Here's how the part is built. I have some questions about the finished solid (model axes, mm). A direction names the side the tool comes from. Round coordinates to 2 decimals unless told otherwise and drop trailing zeros. Write each loop counter-clockwise with the first axis right and the second up, starting at its lowest first coordinate (ties: lowest second). Pieces come first, ordered by that corner, then holes. Notation, with made-up numbers: (-12, -3.5) -> (41, -3.5) arc R22 ccw to (41, 6.5) -> close; hole circle Ø1 at (12.5, 73). An arc over 180 degrees is marked (long way). Put each result on its own line as item: value. Start each with the question number.
1) I want a section at B-B, the plane z = 25. List the corners of the cut face in (x, y) for me.
2) Which directions (+Z, -Z, +X, -X, +Y, -Y) give clear straight access to the entire face, cutting with the end or side of a thin tool? Please do faces 4 (the cylindrical face through (-0.03, 0.24, 35.64)), 5 (the conical face through (0.047, 2.147, 33.856)), 6 (the flat face through (1.9, 0, 33.9)), 7 (the cylindrical face through (-2.539, -1.947, 0.74)), 8 (the flat face through (0, -2.1, 1.5)).
3) I want a section at D-D, the plane y = 2.75. List the corners of the cut face in (x, z) for me, then the cut area to 3 significant figures.
4) Will these pins go through, and if not, where does the flat tip stop? P1, Ø1.5, axis at y = 0.5, z = 33.5, coming from the -X side; P2, Ø3, axis at x = 2, z = 26.5, coming from the -Y side; P3, Ø1.5, axis at y = -0.5, z = 33, coming from the +X side.
5) I want a section at C-C, the plane x = -2.5. List the corners of the cut face in (y, z) for me.
6) If I drill on line 1 along X through (y, z) = (0, 26.5); line 2 along Z through (x, y) = (-2, 1.5); line 3 along Y through (x, z) = (-1.75, 35.5), over which ranges is the centre line in solid material (lowest first)? Write a range as [from, to].
7) I want a section at A-A, the plane x = 0. List the corners of the cut face in (y, z) for me.
8) We'd pull the mould along Z, two halves only. Please class faces 1 (the conical face through (-0.047, -2.147, 33.856)), 2 (the flat face through (0, 0, 36.5)), 3 (the flat face through (-1.9, 0, 33.9)): released by +Z, released by -Z, zero draft, split by the parting line, or undercut.
from build123d import *

# Parameters (mm, degrees)
SKETCH_1_R          = 3.2
EXTRUDE_1_DEPTH     = 1.5
SKETCH_2_R          = 1.9
EXTRUDE_2_DEPTH     = 30
SKETCH_4_R          = 1.9
EXTRUDE_3_DEPTH     = 5
EXTRUDE_3_DRAFT     = -6
SKETCH_5_W          = 1.201314004
SKETCH_5_H          = 17.589809259
CUT_EXTRUDE_4_DEPTH = 17.5
SKETCH_6_R          = 0.8
CUT_EXTRUDE_5_DEPTH = 37.993242626
FILLET_1_R          = 0.2


with BuildPart() as part:
    # Эскиз1 → Вытянуть1 (new body)
    with BuildSketch(Plane.XY):
        Circle(SKETCH_1_R)
    extrude(amount=EXTRUDE_1_DEPTH)

    # Эскиз2 → Вытянуть2 (add)
    with BuildSketch(Plane.XY.offset(1.5)):
        Circle(SKETCH_2_R)
    extrude(amount=EXTRUDE_2_DEPTH)


with BuildPart() as extrude_3_tool:
    # Эскиз4 → Вытянуть3 (with draft: the straight prism first)
    with BuildSketch(Plane.XY.offset(31.5)):
        Circle(SKETCH_4_R)
    extrude(amount=EXTRUDE_3_DEPTH)
    # Вытянуть3: the draft: its side faces are tilted about the plane it starts from
    extrude_3_sides = [extrude_3_tool.faces().sort_by_distance(p)[0] for p in [
        (-1.9, 0, 34),
    ]]
    draft(extrude_3_sides, Plane.XY.offset(31.5), EXTRUDE_3_DRAFT)


with BuildPart() as part_1:
    add(part.part)

    # Вытянуть3: add extrude_3_tool
    add(extrude_3_tool.part)

    # Эскиз5 → Вытянуть4 (cut, symmetric)
    with BuildSketch(Plane(origin=(0, 0, 0), x_dir=(1, 0, 0), z_dir=(0, 1, 0))):
        with Locations((2.500657002, -40.29490463)):
            Rectangle(SKETCH_5_W, SKETCH_5_H)
        with Locations((-2.500657002, -40.29490463)):
            Rectangle(SKETCH_5_W, SKETCH_5_H)
    extrude(amount=CUT_EXTRUDE_4_DEPTH, both=True, mode=Mode.SUBTRACT)

    # Эскиз6 → Вытянуть5 (cut, through all)
    with BuildSketch(Plane.ZY.offset(1.9)):
        with Locations((34.877288216, 0)):
            Circle(SKETCH_6_R)
    extrude(amount=-CUT_EXTRUDE_5_DEPTH, mode=Mode.SUBTRACT)

    # Скругление1
    fillet_1_edges = [part_1.edges().sort_by_distance(p)[0] for p in [
        (0, 2.425521176, 36.5),
        (0, -2.425521176, 36.5),
        (1.9, 0, 36.5),
        (-1.9, 0, 36.5),
    ]]
    fillet(fillet_1_edges, radius=FILLET_1_R)


solid = part_1.part
Findings:
1. outline: circle Ø3.8 at (0, 0)
2. face 4: +X, -X
2. face 5: +Y
2. face 6: +Z, +X, +Y, -Y
2. face 7: +Z, -Z
2. face 8: none
3. outline: (-1.64, 0) -> (1.64, 0) -> (1.64, 1.5) -> (-1.64, 1.5) -> close
3. area: 4.91 mm2
4. P1: stops at x = -1.9
4. P2: stops at y = -1.83
4. P3: stops at x = 1.9
5. outline: (-2, 0) -> (2, 0) -> (2, 1.5) -> (-2, 1.5) -> close
6. line 1: x = [-1.9, 1.9]
6. line 2: z = [0, 1.5]
6. line 3: y = [-1.52, -0.5], [0.5, 1.52]
7. outline: (-3.2, 0) -> (3.2, 0) -> (3.2, 1.5) -> (1.9, 1.5) -> (1.9, 31.5) -> (2.4, 36.28) arc R0.2 ccw to (2.2, 36.5) -> (-2.2, 36.5) arc R0.2 ccw to (-2.4, 36.28) -> (-1.9, 31.5) -> (-1.9, 1.5) -> (-3.2, 1.5) -> close; hole circle Ø1.6 at (0, 34.88)
8. face 1: undercut
8. face 2: released by +Z
8. face 3: zero draft
